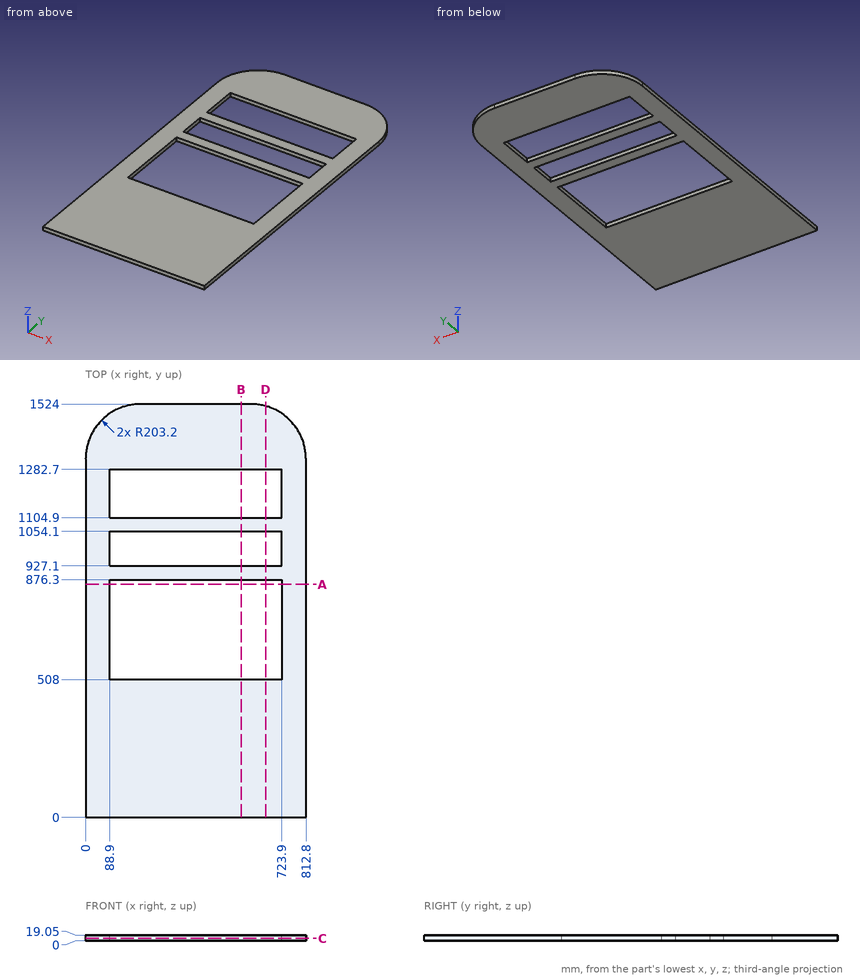
The figure shows three views and two pictorial views of one solid part (mm, origin at its lowest corner). Answer the questions. Give positions to 0.01 mm unless a question says otherwise; leave off trailing zeros. Order: outer loops, then holes, each group sorted by start corner. A loop starts at its lowest first (then second) coordinate and runs counter-clockwise, first axis right, second up. Notation, with made-up numbers: (-33, 74) -> (-29, 74) arc R24 cw to (-29, 96) -> close; hole circle Ø11 at (0, 83.25). An arc over 180 degrees is marked (long way). One line per item, written item: value.
1) Find section C-C, the plane z = 8. Determine the outline of the cut face in (x, y), plus the area to 3 significant figures.
Reported:
outline: (0, 0) -> (812.8, 0) -> (812.8, 1320.8) arc R203.2 ccw to (609.6, 1524) -> (203.2, 1524) arc R203.2 ccw to (0, 1320.8) -> close; hole (88.9, 508) -> (723.9, 508) -> (723.9, 876.3) -> (88.9, 876.3) -> close; hole (88.9, 927.1) -> (723.9, 927.1) -> (723.9, 1054.1) -> (88.9, 1054.1) -> close; hole (88.9, 1104.9) -> (723.9, 1104.9) -> (723.9, 1282.7) -> (88.9, 1282.7) -> close
area: 794,000 mm^2
2) Find the intervals of material crossed by line 1 (Y direction, x = 501.5, z = 6.25); line 2 (X direction, y = 735.5, z = 7.5); line 3 (Y direction, x = 677.5, z = 17.25), in increasing order.
Reported:
line 1: y = 0 to 508, 876.3 to 927.1, 1054.1 to 1104.9, 1282.7 to 1524
line 2: x = 0 to 88.9, 723.9 to 812.8
line 3: y = 0 to 508, 876.3 to 927.1, 1054.1 to 1104.9, 1282.7 to 1512.32
3) Find section D-D, the plane x = 664. Determine the outline of the cut face in (y, z), plus the area to 3 significant figures.
Reported:
outline: (0, 0) -> (508, 0) -> (508, 19.05) -> (0, 19.05) -> close; (876.3, 0) -> (927.1, 0) -> (927.1, 19.05) -> (876.3, 19.05) -> close; (1054.1, 0) -> (1104.9, 0) -> (1104.9, 19.05) -> (1054.1, 19.05) -> close; (1282.7, 0) -> (1516.58, 0) -> (1516.58, 19.05) -> (1282.7, 19.05) -> close
area: 16,100 mm^2
4) Find section A-A, the plane y = 859. Determine the outline of the cut face in (x, z).
Reported:
outline: (0, 0) -> (88.9, 0) -> (88.9, 19.05) -> (0, 19.05) -> close; (723.9, 0) -> (812.8, 0) -> (812.8, 19.05) -> (723.9, 19.05) -> close
5) Find section B-B, the plane x = 573.5. Determine the outline of the cut face in (y, z), plus the area to 3 significant figures.
Reported:
outline: (0, 0) -> (508, 0) -> (508, 19.05) -> (0, 19.05) -> close; (876.3, 0) -> (927.1, 0) -> (927.1, 19.05) -> (876.3, 19.05) -> close; (1054.1, 0) -> (1104.9, 0) -> (1104.9, 19.05) -> (1054.1, 19.05) -> close; (1282.7, 0) -> (1524, 0) -> (1524, 19.05) -> (1282.7, 19.05) -> close
area: 16,200 mm^2
